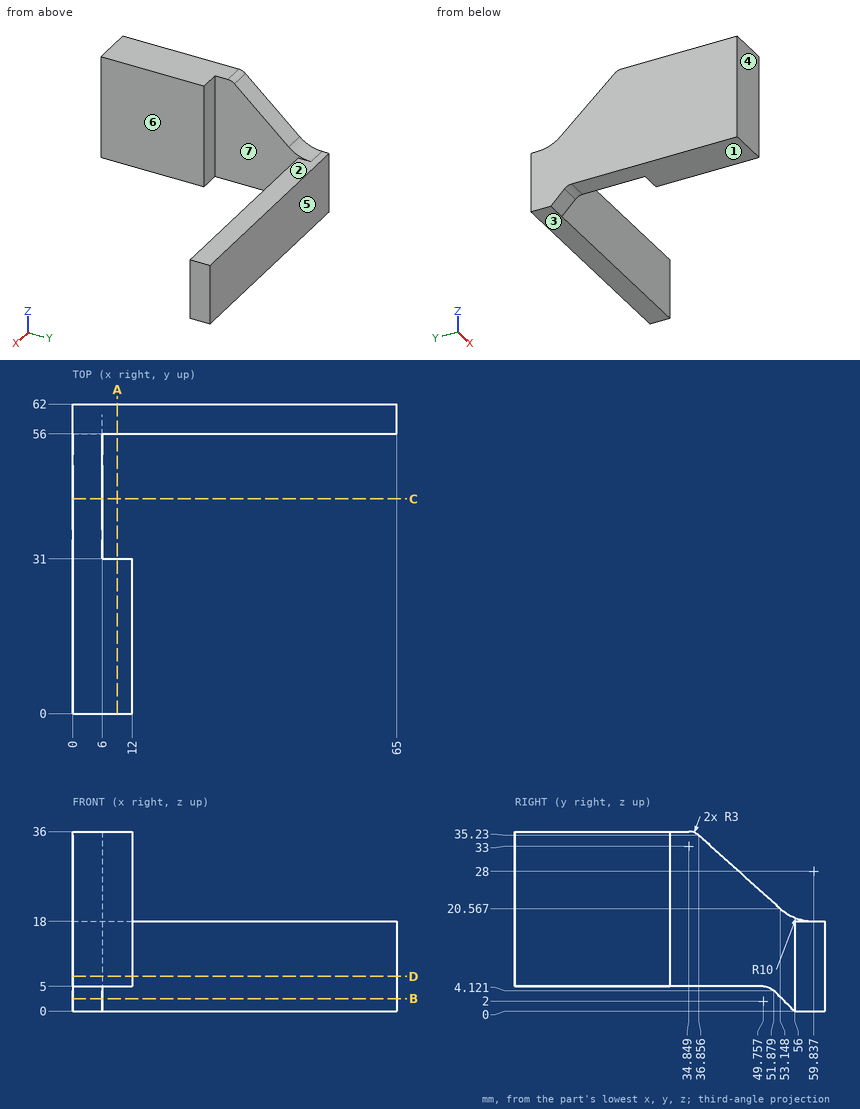
Could you check a few things on this drawing? It's one solid part, dimensions in mm from its lowest x, y, z. A direction names the side the tool comes from. Round coordinates to 2 decimals unless told otherwise and drop trailing zeros. Write each loop counter-clockwise with the first axis right and the second up, starting at its lowest first coordinate (ties: lowest second). Pieces come first, ordered by that corner, then holes. Notation, with made-up numbers: (45, -8) -> (64, -8) arc R29 ccw to (64, 20) -> close; hole circle Ø11 at (-16.75, 66). An arc over 180 degrees is marked (long way). One line per item, written item: value.
1) For the marked faces 1, 2 and 3, which set-ups out of +Z, -Z, +X, -X, +Y, -Y let a thin tool reach every point of the face, with its end or its side?
Filled sheet:
face 1: -Z, +X, -X, -Y
face 2: +Z, +X, +Y
face 3: -Z, +X, -X, +Y, -Y
2) Suppose I cut it at D-D on z = 7. List the corners of the cut face in (x, y) for me, plus the area to 3 significant figures.
Filled sheet:
outline: (0, 0) -> (12, 0) -> (12, 31) -> (6, 31) -> (6, 56) -> (65, 56) -> (65, 62) -> (0, 62) -> close
area: 912 mm2
3) If I drill on line 1 (Y direction, x = 10, z = 13.5); line 2 (X direction, y = 29.5, z = 26.5); line 3 (X direction, y = 43.5, z = 7), over which ranges is the centre line in solid material (lowest first)? Write a range as [from, to].
Filled sheet:
line 1: y = [0, 31], [56, 62]
line 2: x = [0, 12]
line 3: x = [0, 6]
4) Suppose I cut it at A-A on x = 9. List the corners of the cut face in (y, z) for me.
Filled sheet:
outline: (0, 5) -> (31, 5) -> (31, 36) -> (0, 36) -> close; (56, 0) -> (62, 0) -> (62, 18) -> (56, 18) -> close
5) I'm going to push flat-ended pins straight in: pin 1 Ø5 at (x, y) = (23.5, 55) entering from +Z; pin 2 Ø1.8 at (x, z) = (10.5, 20.5) entering from +Y; pin 3 Ø8 at (y, z) = (14.5, 31) entering from +X. Where does each tip first touch, or does it pass through?
Filled sheet:
pin 1: stops at z = 18
pin 2: stops at y = 31
pin 3: stops at x = 12
6) Suppose I cut it at B-B on z = 2.5. List the corners of the cut face in (x, y) for me.
Filled sheet:
outline: (0, 53.5) -> (6, 53.5) -> (6, 56) -> (65, 56) -> (65, 62) -> (0, 62) -> close
7) Suppose I cut it at C-C on y = 43. List the corners of the cut face in (x, z) for me.
Filled sheet:
outline: (0, 5) -> (6, 5) -> (6, 29.7) -> (0, 29.7) -> close
8) We'd pull the mould along Y, two halves only. Please class the marked faces 4, 5, 6 and 7: released by +Y, released by -Y, zero draft, split by the parting line, or undercut.
Filled sheet:
face 4: released by -Y
face 5: released by +Y
face 6: zero draft
face 7: undercut
